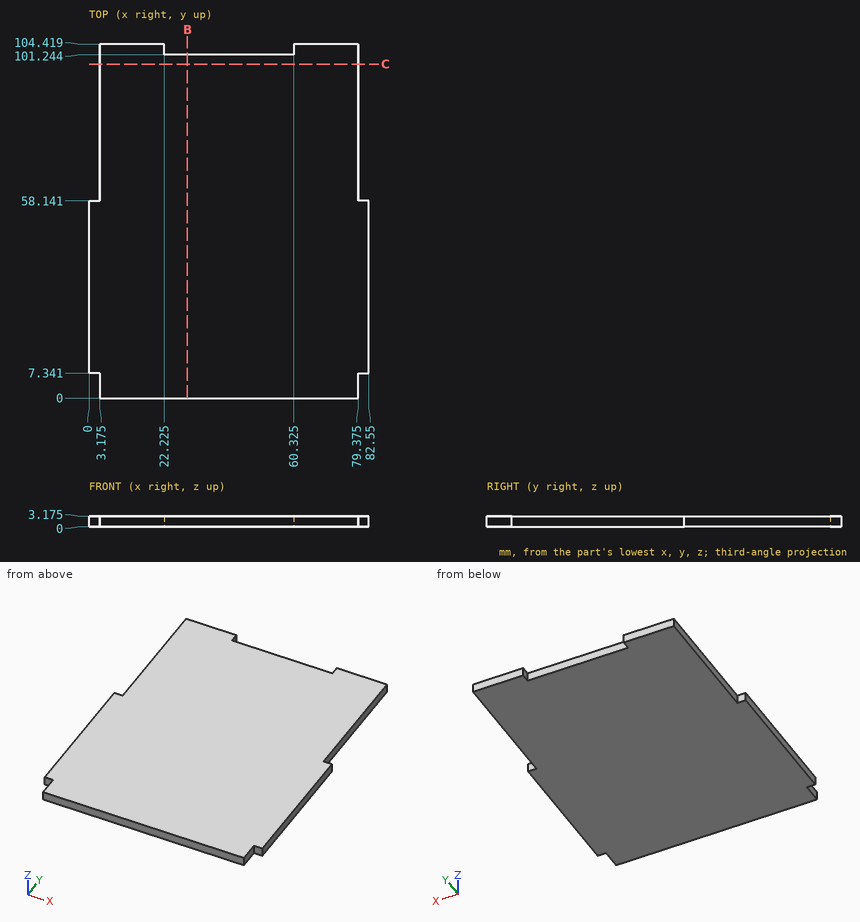
Drawing for the job (mm, zero at the part's lowest x, y, z). Give positions to 0.01 mm unless a question says otherwise; leave off trailing zeros. Loops run counter-clockwise (first coordinate to the right, second up) from the corner with the lowest first, then second, coordinate; pieces in that order, holes last. Notation, with made-up numbers: (80.25, 84.25) - (134.25, 84.25) arc R22 cw to (134.25, 98.25) - close; hole circle Ø6 at (73.5, 35.5). An arc over 180 degrees is marked (long way). Write item = value, one per line. Start each with the question number.
1) Band-saw the part on B-B on x = 29. Give the cut face in (y, z) (1 decimal).
2) Drop flat-ended pins along their axis: pin 1 Ø1 at (y, z) = (75, 1) entering from +X (3 decimals); pin 2 Ø1 at (x, z) = (1, 1.5) entering from +Y; pin 3 Ø1 at (x, z) = (39.5, 2) entering from +Y. Give the stop position or say it passes through.
3) Probe probe 1 along Y at (x, z) = (22.5, 1.25) (1 decimal); probe 2 along X at (y, z) = (92, 2.3) (1 decimal). List the from-to ranges inside material, lowest first. Write a range as from..to.
4) Band-saw the part on C-C on y = 98.5. Give the cut face in (x, z) (1 decimal).
Final values:
q1.outline = (0, 0) - (101.2, 0) - (101.2, 3.2) - (0, 3.2) - close
q2.pin_1 = 79.375
q2.pin_2 = 58.14
q2.pin_3 = 101.24
q3.probe_1 = 0..101.2
q3.probe_2 = 3.2..79.4
q4.outline = (3.2, 0) - (79.4, 0) - (79.4, 3.2) - (3.2, 3.2) - close
